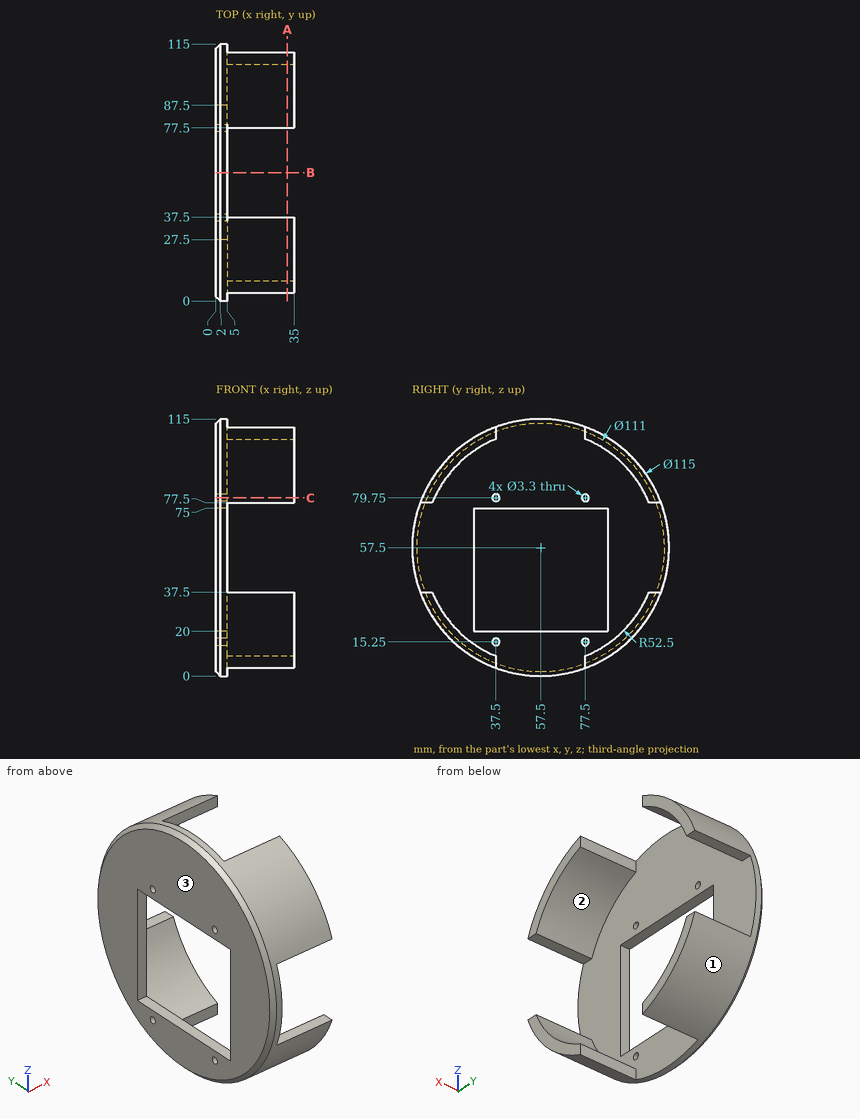
Geometry check sheet. Reference: drawing and pictorial views, mm from the part's lowest x, y, z. Round coordinates to 2 decimals unless told otherwise and drop trailing zeros. Write each loop counter-clockwise with the first axis right and the second up, starting at its lowest first coordinate (ties: lowest second). Pieces come first, ordered by that corner, then holes. Notation, with made-up numbers: (58, 17) -> (111, 17) arc R35 cw to (111, 51) -> close; hole circle Ø4 at (-14.75, 68.25). An arc over 180 degrees is marked (long way). Put each result on its own line as item: value.
1) Release check for a two-part mould opening along Z. For the marked faces 1, 2 and 3 record: pulls with the +Z half, pulls with the -Z half, needs draft (parallel to the pull), parting line crosses it, or undercut.
Recorded:
face 1: parting line crosses it
face 2: undercut
face 3: needs draft
2) Depth check by flat-ended pin: P1, Ø1.6, axis at x = 25, y = 108, coming from the +Z side; P2, Ø4.5, axis at x = 19, y = 6, coming from the -Z side; P3, Ø4.5, axis at x = 24.5, z = 7.5, coming from the -Y side; P4, Ø10, axis at x = 13, z = 46.5, coming from the -Y side. Enter the tip coordinate at first touch or a pass-through.
Recorded:
P1: stops at z = 86.42
P2: stops at z = 27.82
P3: stops at y = 25.47
P4: passes through
3) Cross-section at B-B, the plane y = 57.5. Enter the section's corners in (x, z), plus the area to 3 significant figures.
Recorded:
outline: (0, 2) -> (2, 0) -> (5, 0) -> (5, 20) -> (0, 20) -> close; (0, 75) -> (5, 75) -> (5, 115) -> (2, 115) -> (0, 113) -> close
area: 296 mm2
4) Thickness scan on probe 1 along Z at (x, y) = (2.85, 77.5); probe 2 along Z at (x, y) = (2, 37); probe 3 along Y at (x, z) = (2, 79). Record the ranges inside material, lowest first. Write a range as from..to.
Recorded:
probe 1: z = 3.59..13.6, 16.9..20, 75..78.1, 81.4..111.41
probe 2: z = 3.78..13.68, 16.82..20, 75..78.18, 81.32..111.22
probe 3: y = 4.17..36.03, 38.97..76.03, 78.97..110.83
5) Cross-section at A-A, the plane x = 32. Enter the section's corners in (y, z), plus the area to 3 significant figures.
Recorded:
outline: (3.59, 37.5) arc R57.5 ccw to (37.5, 3.59) -> (37.5, 8.96) arc R52.5 cw to (8.96, 37.5) -> close; (3.59, 77.5) -> (8.96, 77.5) arc R52.5 cw to (37.5, 106.04) -> (37.5, 111.41) arc R57.5 ccw to start; (77.5, 3.59) arc R57.5 ccw to (111.41, 37.5) -> (106.04, 37.5) arc R52.5 cw to (77.5, 8.96) -> close; (77.5, 106.04) arc R52.5 cw to (106.04, 77.5) -> (111.41, 77.5) arc R57.5 ccw to (77.5, 111.41) -> close
area: 909 mm2
6) Cross-section at C-C, the plane z = 79.75. Give the number of separate pieces and of enclosed holes in the cut face, plus the area to 3 significant figures.
Recorded:
separate pieces: 3
enclosed holes: 0
area: 821 mm2
